Input: part model. Units: mm. Frame: model coordinates. A direction names the side the tool comes from. Coordinates: 2 decimals unless noted, no trailing zeros. Order: outer loops, then holes, each group sorted by start corner. A loop starts at its lowest first (then second) coordinate and runs counter-clockwise, first axis right, second up.
from build123d import *

# Parameters (mm, degrees)
F1_DEPTH = 70
F3_DEPTH = 8
F5_DEPTH = 9
F6_R     = 1.875
F7_DEPTH = 9


# Not quite as in the source:
# - a feature names something its author has since deleted; it is built from what else it names


with BuildPart() as f1:
    # F0 (on Right) → F1 (new body)
    with BuildSketch(Plane.YZ):
        Polygon((15.9777059274, -37.1211464703), (15.9777059274, 43.8788535297), (9.9777059274, 43.8788535297), (9.9777059274, -31.1211464703), (5.4777059274, -31.1211464703), (5.4777059274, -16.1211464703), (-0.5222940726, -16.1211464703), (-0.5222940726, -37.1211464703), align=None)
    extrude(amount=F1_DEPTH)

    # F2 (on face) → F3 (join)
    with BuildSketch(Plane.YZ.offset(70)):
        with BuildLine():
            Line((12.9777059274, 33.8788535297), (12.9777059274, 35.3788535297))
            ThreePointArc((12.9777059274, 35.3788535297), (11.4777059274, 33.8788535297), (12.9777059274, 32.3788535297))
            Line((12.9777059274, 32.3788535297), (12.9777059274, 33.8788535297))
        make_face()
        with BuildLine():
            ThreePointArc((12.9777059274, 32.3788535297), (14.0383660992, 32.8181933579), (14.4777059274, 33.8788535297))
            ThreePointArc((14.4777059274, 33.8788535297), (14.0383660992, 34.9395137015), (12.9777059274, 35.3788535297))
            Line((12.9777059274, 35.3788535297), (12.9777059274, 33.8788535297))
            Line((12.9777059274, 33.8788535297), (12.9777059274, 32.3788535297))
        make_face()
        with BuildLine():
            Line((12.9777059274, 13.8788535297), (12.9777059274, 15.3178830066))
            ThreePointArc((12.9777059274, 15.3178830066), (11.4636811456, 13.8179485729), (12.9777059274, 12.3180141391))
            Line((12.9777059274, 12.3180141391), (12.9777059274, 13.8788535297))
        make_face()
        with BuildLine():
            ThreePointArc((14.4636811456, 13.8179485729), (14.0292882901, 14.8736385906), (12.9777059274, 15.3178830066))
            Line((12.9777059274, 15.3178830066), (12.9777059274, 13.8788535297))
            Line((12.9777059274, 13.8788535297), (12.9777059274, 12.3180141391))
            ThreePointArc((12.9777059274, 12.3180141391), (14.0292882901, 12.7622585551), (14.4636811456, 13.8179485729))
        make_face()
        with BuildLine():
            Line((12.9777059274, -7.1211464703), (12.9777059274, -5.7047228841))
            ThreePointArc((12.9777059274, -5.7047228841), (11.5072213267, -7.2044324698), (12.9777059274, -8.7041420554))
            Line((12.9777059274, -8.7041420554), (12.9777059274, -7.1211464703))
        make_face()
        with BuildLine():
            ThreePointArc((14.5072213267, -7.2044324698), (14.0573943841, -6.1333878631), (12.9777059274, -5.7047228841))
            Line((12.9777059274, -5.7047228841), (12.9777059274, -7.1211464703))
            Line((12.9777059274, -7.1211464703), (12.9777059274, -8.7041420554))
            ThreePointArc((12.9777059274, -8.7041420554), (14.0573943841, -8.2754770764), (14.5072213267, -7.2044324698))
        make_face()
        with BuildLine():
            ThreePointArc((12.9777059274, -25.6469734003), (11.473965778, -27.1469687374), (12.9777059274, -28.6469640745))
            Line((12.9777059274, -28.6469640745), (12.9777059274, -27.1211464703))
            Line((12.9777059274, -27.1211464703), (12.9777059274, -25.6469734003))
        make_face()
        with BuildLine():
            Line((12.9777059274, -27.1211464703), (12.9777059274, -28.6469640745))
            ThreePointArc((12.9777059274, -28.6469640745), (14.035947469, -28.2063057413), (14.473965778, -27.1469687374))
            ThreePointArc((14.473965778, -27.1469687374), (14.035947469, -26.0876317334), (12.9777059274, -25.6469734003))
            Line((12.9777059274, -25.6469734003), (12.9777059274, -27.1211464703))
        make_face()
    extrude(amount=F3_DEPTH)

    # F4 (on face) → F5 (cut)
    with BuildSketch(Plane(origin=(0, 0, 0), x_dir=(0, -1, 0), z_dir=(-1, 0, 0))):
        with BuildLine():
            ThreePointArc((-12.9777059274, 32.0038535297), (-11.6518807127, 32.553028315), (-11.1027059274, 33.8788535297))
            ThreePointArc((-11.1027059274, 33.8788535297), (-11.6518807127, 35.2046787444), (-12.9777059274, 35.7538535297))
            Line((-12.9777059274, 35.7538535297), (-12.9777059274, 33.8788535297))
            Line((-12.9777059274, 33.8788535297), (-12.9777059274, 32.0038535297))
        make_face()
        with BuildLine():
            Line((-12.9777059274, 33.8788535297), (-12.9777059274, 35.7538535297))
            ThreePointArc((-12.9777059274, 35.7538535297), (-14.8527059274, 33.8788535297), (-12.9777059274, 32.0038535297))
            Line((-12.9777059274, 32.0038535297), (-12.9777059274, 33.8788535297))
        make_face()
        with BuildLine():
            ThreePointArc((-11.1027059274, 13.8788535297), (-11.6518807127, 15.2046787444), (-12.9777059274, 15.7538535297))
            ThreePointArc((-12.9777059274, 15.7538535297), (-14.3035311422, 12.553028315), (-11.1027059274, 13.8788535297))
        make_face()
        with BuildLine():
            ThreePointArc((-11.1027059274, -7.1211464703), (-14.3035311422, -5.7953212556), (-12.9777059274, -8.9961464703))
            ThreePointArc((-12.9777059274, -8.9961464703), (-11.6518807127, -8.446971685), (-11.1027059274, -7.1211464703))
        make_face()
        with BuildLine():
            ThreePointArc((-12.9777059274, -25.2461464703), (-14.8527059274, -27.1211464703), (-12.9777059274, -28.9961464703))
            Line((-12.9777059274, -28.9961464703), (-12.9777059274, -27.1211464703))
            Line((-12.9777059274, -27.1211464703), (-12.9777059274, -25.2461464703))
        make_face()
        with BuildLine():
            Line((-12.9777059274, -27.1211464703), (-12.9777059274, -28.9961464703))
            ThreePointArc((-12.9777059274, -28.9961464703), (-11.6518807127, -28.446971685), (-11.1027059274, -27.1211464703))
            ThreePointArc((-11.1027059274, -27.1211464703), (-11.6518807127, -25.7953212556), (-12.9777059274, -25.2461464703))
            Line((-12.9777059274, -25.2461464703), (-12.9777059274, -27.1211464703))
        make_face()
    extrude(amount=-F5_DEPTH, mode=Mode.SUBTRACT)

    # F6 (on face) → F7 (cut)
    with BuildSketch(Plane(origin=(0, 15.9777059274, 0), x_dir=(-1, 0, 0), z_dir=(0, 1, 0))):
        with Locations((-55, -34.1211464703)):
            Circle(F6_R)
        with Locations((-35, -34.1211464703)):
            Circle(F6_R)
        with Locations((-15, -34.1211464703)):
            Circle(F6_R)
    extrude(amount=-F7_DEPTH, mode=Mode.SUBTRACT)


solid = f1.part
Item 1: Cut plane D-D on y = 4.5. Return loops of the section in (x, z).
Response values:
outline: (0, -37.12) - (70, -37.12) - (70, -16.12) - (0, -16.12) - close
Item 2: Draft query along X for faces 1 (the face through (78, 13, -27)), 2 (the face through (16.873, 11.541, -34.039)), 3 (the face through (0, 11, -5)), 4 (the face through (35, 8, -31.121)). Return one class per face: pulls with the +X half, pulls with the -X half, needs draft (parallel to the pull), parting line crosses it, or undercut.
Response values:
face 1: pulls with the +X half
face 2: undercut
face 3: pulls with the -X half
face 4: needs draft
Item 3: Ray query, probe 1 along Y at (x, z) = (27, -17); probe 2 along Z at (x, y) = (15, 11); probe 3 along Y at (x, z) = (23, 26.5). Return the intervals inside material, ascending.
Response values:
probe 1: y = -0.52 to 5.48, 9.98 to 15.98
probe 2: z = -37.12 to -36, -32.25 to 43.88
probe 3: y = 9.98 to 15.98
Item 4: Access query for faces 5 (the face through (9, 13, 34)), 6 (the face through (35, -0.522, -26)), 7 (the face through (35, 13, 43.879)), 8 (the face through (35, 6.978, -34)), 9 (the face through (35, 3, -16.121)). Directions: +Z, -Z, +X, -X, +Y, -Y. A direction counts if a zero-diameter tool reaches every point of the face in a straight line with its end or side. Return the directions, or none.
Response values:
face 5: -X
face 6: +Z, -Z, +X, -X, -Y
face 7: +Z, +X, -X, +Y, -Y
face 8: +Y
face 9: +Z, +X, -X, -Y
Item 5: Cut plane A-A on x = 55. Return loops of the section in (y, z).
Response values:
outline: (-0.52, -37.12) - (15.98, -37.12) - (15.98, -36) - (6.98, -36) - (6.98, -32.25) - (15.98, -32.25) - (15.98, 43.88) - (9.98, 43.88) - (9.98, -31.12) - (5.48, -31.12) - (5.48, -16.12) - (-0.52, -16.12) - close
Item 6: Cut plane B-B on z = 25. Return loops of the section in (x, y), then the cut area to 3 significant figures.
Response values:
outline: (0, 9.98) - (70, 9.98) - (70, 15.98) - (0, 15.98) - close
area: 420 mm2
Item 7: Cut plane C-C on x = 68. Return loops of the section in (y, z).
Response values:
outline: (-0.52, -37.12) - (15.98, -37.12) - (15.98, 43.88) - (9.98, 43.88) - (9.98, -31.12) - (5.48, -31.12) - (5.48, -16.12) - (-0.52, -16.12) - close
Item 8: Pin query (flat end, axial travel): pin 1 Ø1.1 at (x, z) = (55, -34.5) entering from +Y; pin 2 Ø4 at (x, y) = (32, 4.5) entering from +Z; pin 3 Ø12 at (x, z) = (67, -6) entering from -Y. Return the tip coordinate at first contact, or that it passes through.
Response values:
pin 1: stops at y = 6.98
pin 2: stops at z = -16.12
pin 3: stops at y = 9.98
